Could you check a few things on this model? Use its own coordinates, in mm. Face numbers are marked on the shaded views. A direction names the side the tool comes from. Round coordinates to 2 decimals unless told otherwise and drop trailing zeros. Loops run counter-clockwise (first coordinate to the right, second up) from the corner with the lowest first, then second, coordinate; pieces in that order, holes last. Notation, with made-up numbers: (49, 37.5) - (97, 37.5) arc R22 cw to (97, 72.5) - close; hole circle Ø1 at (33.5, 32). An arc over 180 degrees is marked (long way). Answer as CSV lines item,"result". Start each with the question number.
1) Suppose I cut it at A-A, the plane z = -185. Write out the boundary of the cut face in (x, y).
2) Suppose I cut it at B-B, the plane x = -230. Write out the boundary of the cut face in (y, z), then the cut area to 3 significant figures.
3) Please list where these lines run through material, in increasing order: line 1 along X through (y, z) = (-601, 0); line 2 along Y through (x, z) = (-164, 104); line 3 along Z through (x, y) = (-150, -602.25).
4) Suppose I cut it at C-C, the plane y = -266.5. Write out the boundary of the cut face in (x, z), then the cut area to 3 significant figures.
5) Which directions (+Z, -Z, +X, -X, +Y, -Y) give clear straight access to the entire face, cutting with the end or side of a thin tool? Please do the marked faces 5, 6 and 7.
6) Suppose I cut it at D-D, the plane z = 52.5. Write out the boundary of the cut face in (x, y).
7) We'd pull the mould along Y, two halves only. Please class the marked faces 1, 2, 3 and 4: pulls with the +Y half, pulls with the -Y half, needs draft (parallel to the pull), parting line crosses it, or undercut.
8) I'm going to push flat-ended pins straight in: pin 1 Ø5 at (x, y) = (206, -320) entering from +Z; pin 2 Ø5 at (x, z) = (-148, 1) entering from -Y; pin 3 Ø1 at (x, y) = (18.5, -133.5) entering from +Z. Where does each tip first touch, or does it pass through?
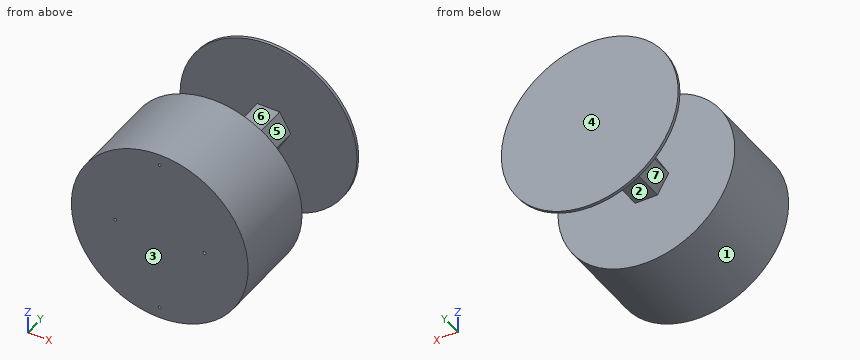
```python
from build123d import *

# Parameters (mm, degrees)
SKETCH1_R           = 297.326212148
BOSS_EXTRUDE1_DEPTH = 10
BOSS_EXTRUDE2_DEPTH = 305
BOSS_EXTRUDE3_START = 300
SKETCH3_R           = 297.326212148
BOSS_EXTRUDE3_DEPTH = 300
SKETCH5_R           = 5
CUT_EXTRUDE1_DEPTH  = 10
SKETCH6_R           = 5
CUT_EXTRUDE2_DEPTH  = 10


with BuildPart() as part:
    # Sketch1 → Boss-Extrude1 (new body)
    with BuildSketch(Plane(origin=(0, 0, 0), x_dir=(1, 0, 0), z_dir=(0, 1, 0))):
        with Locations(Location((0, 0, 0), (0, 0, 270))):
            Circle(SKETCH1_R)
    extrude(amount=BOSS_EXTRUDE1_DEPTH)

    # Sketch2 → Boss-Extrude2 (add)
    with BuildSketch(Plane.XZ):
        Polygon((75, 0), (37.5, 64.951905284), (-37.5, 64.951905284), (-75, 0), (-37.5, -64.951905284), (37.5, -64.951905284), align=None)
    extrude(amount=BOSS_EXTRUDE2_DEPTH)

    # Sketch3 → Boss-Extrude3 (add)
    with BuildSketch(Plane.XZ.offset(305).offset(BOSS_EXTRUDE3_START)):
        with Locations(Location((0, 0, 0), (0, 0, 90))):
            Circle(SKETCH3_R)
    extrude(amount=-BOSS_EXTRUDE3_DEPTH)

    # Sketch5 → Cut-Extrude1 (cut)
    with BuildSketch(Plane.XZ.offset(605)):
        with Locations(Location((150, 0, 0), (0, 0, 270))):
            Circle(SKETCH5_R)
        with Locations(Location((-150, 0, 0), (0, 0, 90))):
            Circle(SKETCH5_R)
    extrude(amount=-CUT_EXTRUDE1_DEPTH, mode=Mode.SUBTRACT)

    # Sketch6 → Cut-Extrude2 (cut)
    with BuildSketch(Plane.XZ.offset(605)):
        with Locations(Location((0, 259.826212148, 0), (0, 0, 270))):
            Circle(SKETCH6_R)
        with Locations(Location((0, -259.826212148, 0), (0, 0, 90))):
            Circle(SKETCH6_R)
    extrude(amount=-CUT_EXTRUDE2_DEPTH, mode=Mode.SUBTRACT)


solid = part.part
```
Filled sheet:
1,outline,"(-232.76, -605) - (232.76, -605) - (232.76, -305) - (-232.76, -305) - close; (-232.76, 0) - (232.76, 0) - (232.76, 10) - (-232.76, 10) - close"
2,outline,"(-605, -188.42) - (-305, -188.42) - (-305, 188.42) - (-605, 188.42) - close; (0, -188.42) - (10, -188.42) - (10, 188.42) - (0, 188.42) - close"
2,area,"117,000 mm²"
3,line 1,"-297.33 to -155, -145 to 145, 155 to 297.33"
3,line 2,"-605 to -305, 0 to 10"
3,line 3,"-256.72 to -5, 5 to 256.72"
4,outline,"(-75, 0) - (-37.5, -64.95) - (37.5, -64.95) - (75, 0) - (37.5, 64.95) - (-37.5, 64.95) - close"
4,area,"14,600 mm²"
5,face 5,"+Z, +X"
5,face 6,"+Z, +X, -X"
5,face 7,"-Z, -X"
6,outline,"(-292.65, -605) - (292.65, -605) - (292.65, -305) - (44.69, -305) - (44.69, 0) - (292.65, 0) - (292.65, 10) - (-292.65, 10) - (-292.65, 0) - (-44.69, 0) - (-44.69, -305) - (-292.65, -305) - close"
7,face 1,"needs draft"
7,face 2,"undercut"
7,face 3,"pulls with the -Y half"
7,face 4,"pulls with the +Y half"
8,pin 1,"z = 216.77"
8,pin 2,"y = -595"
8,pin 3,"z = 64.95"
